Design review of the part built by this model. Coordinates are the model's own, in mm. A direction names the side the tool comes from. Round coordinates to 2 decimals unless told otherwise and drop trailing zeros. Order: outer loops, then holes, each group sorted by start corner. A loop starts at its lowest first (then second) coordinate and runs counter-clockwise, first axis right, second up.
from build123d import *


with BuildPart() as part:
    # Sketch2 → Revolve1 (revolve)
    with BuildSketch(Plane(origin=(0, 0, 0), x_dir=(0, 0, -1), z_dir=(1, 0, 0))):
        with BuildLine():
            Line((6.35, 1.5875), (0, 1.5875))
            Line((0, 1.5875), (0, 3.3274))
            Line((0, 3.3274), (-0.508, 3.3274))
            ThreePointArc((-0.508, 3.3274), (-0.823736431, 2.514400819), (-1.016, 1.6637))
            Line((-1.016, 1.6637), (-1.016, 0.89296875))
            Line((-1.016, 0.89296875), (0, 0.89296875))
            Line((0, 0.89296875), (0.635, 0.89296875))
            Line((0.635, 0.89296875), (0.635, 0))
            Line((0.635, 0), (6.35, 0))
            Line((6.35, 0), (6.35, 1.5875))
        make_face()
    revolve(axis=Axis((0, 0, -6.35), (0, 0, 1)))


solid = part.part
1) For faces 4 (the face through (3.25, -0.72, 0.26)), 5 (the face through (-2, -1, 0)), 6 (the face through (-0.039, -0.892, 0.179)), list the 3-axis set-ups (+Z, -Z, +X, -X, +Y, -Y) from which the entire face can be reached by the end or side of a thin tool; tool diameter is ignored.
Results:
face 4: +Z, -Z
face 5: -Z
face 6: +Z
2) Take a section at B-B on z = -5. Give the boundary of the cut face in (x, y) (1 decimal).
Results:
outline: circle Ø3.2 at (0, 0)
3) Clearance check with flat-ended pins moving along their axes: P1, Ø1.5, axis at y = -1.5, z = 0, coming from the +X side; P2, Ø2, axis at x = -1.5, z = 0, coming from the +Y side; P3, Ø2, axis at x = -0.5, y = 0, coming from the +Z side; P4, Ø1.5, axis at x = -2, z = -3.5, coming from the +Y side. State where each tip first meets the part, or that it passes through.
Results:
P1: stops at x = 3.24
P2: stops at y = 3.29
P3: stops at z = 1.02
P4: stops at y = 0.98
4) To check wall thickness, follow line 1 along Y through (x, z) = (0, 0.15); line 2 along X through (y, z) = (0, -0.3). State the ranges of each line that lie inside material, in increasing order.
Results:
line 1: y = -3.33 to -0.89, 0.89 to 3.33
line 2: x = -1.59 to -0.89, 0.89 to 1.59
5) Take a section at A-A on z = -0.25. Give the boundary of the cut face in (x, y) (1 decimal).
Results:
outline: circle Ø3.2 at (0, 0); hole circle Ø1.8 at (0, 0)
6) The part is to be moulded in two halves that separate along X. For faces 1 (the face through (1, 1, 1.016)), 2 (the face through (1.55, -0.34, -3.13)), 3 (the face through (0, 0, -0.635)), say which applies: released by +X, released by -X, zero draft, split by the parting line, or undercut.
Results:
face 1: zero draft
face 2: split by the parting line
face 3: undercut
